Geometry check sheet. Reference: the model listing, model coordinates, mm. Give positions to 0.01 mm unless a question says otherwise; leave off trailing zeros. Write each loop counter-clockwise with the first axis right and the second up, starting at its lowest first coordinate (ties: lowest second). Pieces come first, ordered by that corner, then holes. Notation, with made-up numbers: (25, 26.25) -> (30, 26.25) arc R35 ccw to (30, 63.25) -> close; hole circle Ø9 at (-39.5, 18). An arc over 180 degrees is marked (long way). One line per item, written item: value.
from build123d import *

# Parameters (mm, degrees)
F0_R     = 1.5
F1_DEPTH = 3
F3_R     = 2.75
F4_DEPTH = 381
F6_R     = 5
F7_R     = 2.5
F8_DEPTH = 25


with BuildPart() as f1:
    # F0 (on Front) → F1 (new body)
    with BuildSketch(Plane.XZ):
        with BuildLine():
            Line((12.5, -12.5), (12.5, 0))
            ThreePointArc((12.5, 0), (12.4899799325, -0.5004011242), (12.4599357944, -1))
            ThreePointArc((12.4599357944, -1), (0, -12.5), (-12.4599357944, -1))
            ThreePointArc((-12.4599357944, -1), (-12.4899799325, -0.5004011242), (-12.5, 0))
            Line((-12.5, 0), (-12.5, -67.8362422814))
            Line((-12.5, -67.8362422814), (12.5, -67.8362422814))
            Line((12.5, -67.8362422814), (12.5, -59.3175111059))
            Line((12.5, -59.3175111059), (12.5, -12.5))
        make_face()
        Polygon((12.5, 12.5), (12.5, 0), (12.5, -12.5), (26.5, -12.5), (26.5, 12.5), align=None)
        with BuildLine():
            ThreePointArc((12.4599357944, 1), (12.4899799325, 0.5004011242), (12.5, 0))
            Line((12.5, 0), (12.5, 12.5))
            Line((12.5, 12.5), (0, 12.5))
            ThreePointArc((0, 12.5), (8.4779124789, 9.1855865354), (12.4599357944, 1))
        make_face()
        with BuildLine():
            Line((12.4599357944, -1), (12.4599357944, 1))
            ThreePointArc((12.4599357944, 1), (8.4779124789, 9.1855865354), (0, 12.5))
            ThreePointArc((0, 12.5), (-8.4779124789, 9.1855865354), (-12.4599357944, 1))
            Line((-12.4599357944, 1), (-12.4599357944, -1))
            ThreePointArc((-12.4599357944, -1), (0, -12.5), (12.4599357944, -1))
        make_face()
        Circle(F0_R, mode=Mode.SUBTRACT)
        with BuildLine():
            ThreePointArc((-12.4599357944, 1), (-8.4779124789, 9.1855865354), (0, 12.5))
            Line((0, 12.5), (-12.5, 12.5))
            Line((-12.5, 12.5), (-12.5, 0))
            ThreePointArc((-12.5, 0), (-12.4899799325, 0.5004011242), (-12.4599357944, 1))
        make_face()
        with BuildLine():
            ThreePointArc((-12.5, 0), (-12.4899799325, -0.5004011242), (-12.4599357944, -1))
            Line((-12.4599357944, -1), (-12.4599357944, 1))
            ThreePointArc((-12.4599357944, 1), (-12.4899799325, 0.5004011242), (-12.5, 0))
        make_face()
        Circle(F0_R)
    extrude(amount=F1_DEPTH)

    # F3 (on face) → F4 (cut, symmetric)
    with BuildSketch(Plane.XZ.offset(3)):
        Circle(F3_R)
    extrude(amount=F4_DEPTH, both=True, mode=Mode.SUBTRACT)

    # F6
    f6_edges = [f1.edges().sort_by_distance(p)[0] for p in [
        (12.5, -1.5, -67.836242),
        (-12.5, -1.5, -67.836242),
        (-12.5, -1.5, 12.5),
        (12.5, -1.5, -12.5),
        (26.5, -1.5, -12.5),
        (26.5, -1.5, 12.5),
    ]]
    fillet(f6_edges, radius=F6_R)

    # F7 (on face) → F8 (cut)
    with BuildSketch(Plane.XZ.offset(3)):
        with Locations((14, 0)):
            Circle(F7_R)
        with BuildLine():
            Line((12.4599357944, -1), (12.4599357944, 1))
            ThreePointArc((12.4599357944, 1), (12.5, 0), (12.4599357944, -1))
        make_face(mode=Mode.SUBTRACT)
    extrude(amount=-F8_DEPTH, mode=Mode.SUBTRACT)


solid = f1.part
1) Sectioned sample at A-A on x = 0. Record the cut outline in (y, z), plus the area to 3 significant figures.
Verdict:
outline: (-3, -67.84) -> (0, -67.84) -> (0, -2.75) -> (-3, -2.75) -> close; (-3, 2.75) -> (0, 2.75) -> (0, 12.5) -> (-3, 12.5) -> close
area: 225 mm^2
2) Scan lines: probe 1 along X at (y, z) = (-2.3, -54); probe 2 along Z at (x, y) = (-1.5, -0.5); probe 3 along Z at (x, y) = (14, -2.4). Record each from-to range of solid material in increasing order.
Verdict:
probe 1: -12.5 to 12.5
probe 2: -67.84 to -2.3, 2.3 to 12.5
probe 3: -13.93 to -2.5, 2.5 to 12.5
3) Depth check by flat-ended pin: pin 1 Ø1.5 at (y, z) = (-1.5, -35.5) entering from +X. Enter the tip coordinate at first touch or a pass-through.
Verdict:
pin 1: x = 12.5
4) Sectioned sample at C-C on y = -1.65. Record the cut outline in (x, z).
Verdict:
outline: (-12.5, -62.84) arc R5 ccw to (-7.5, -67.84) -> (7.5, -67.84) arc R5 ccw to (12.5, -62.84) -> (12.5, -17.5) arc R5 cw to (17.5, -12.5) -> (21.5, -12.5) arc R5 ccw to (26.5, -7.5) -> (26.5, 7.5) arc R5 ccw to (21.5, 12.5) -> (-7.5, 12.5) arc R5 ccw to (-12.5, 7.5) -> close; hole circle Ø5.5 at (0, 0); hole circle Ø5 at (14, 0)
5) Sectioned sample at D-D on z = -43.5. Record the cut outline in (x, y), plus the area to 3 significant figures.
Verdict:
outline: (-12.5, -3) -> (12.5, -3) -> (12.5, 0) -> (-12.5, 0) -> close
area: 75.0 mm^2
6) Mould release check, pull along Z, two halves, no side actions. Record for faces 1 (the cylindrical face through (11.5, -1.5, 0.1)), 2 (the flat face through (12.5, -1, -40)), 3 (the flat face through (19, -1, -12.5)): released by +Z, released by -Z, zero draft, split by the parting line, or undercut.
Verdict:
face 1: undercut
face 2: zero draft
face 3: released by -Z
7) Sectioned sample at B-B on z = 0. Record the cut outline in (x, y), plus the area to 3 significant figures.
Verdict:
outline: (-12.5, -3) -> (-2.75, -3) -> (-2.75, 0) -> (-12.5, 0) -> close; (2.75, -3) -> (11.5, -3) -> (11.5, 0) -> (2.75, 0) -> close; (16.5, -3) -> (26.5, -3) -> (26.5, 0) -> (16.5, 0) -> close
area: 85.5 mm^2
